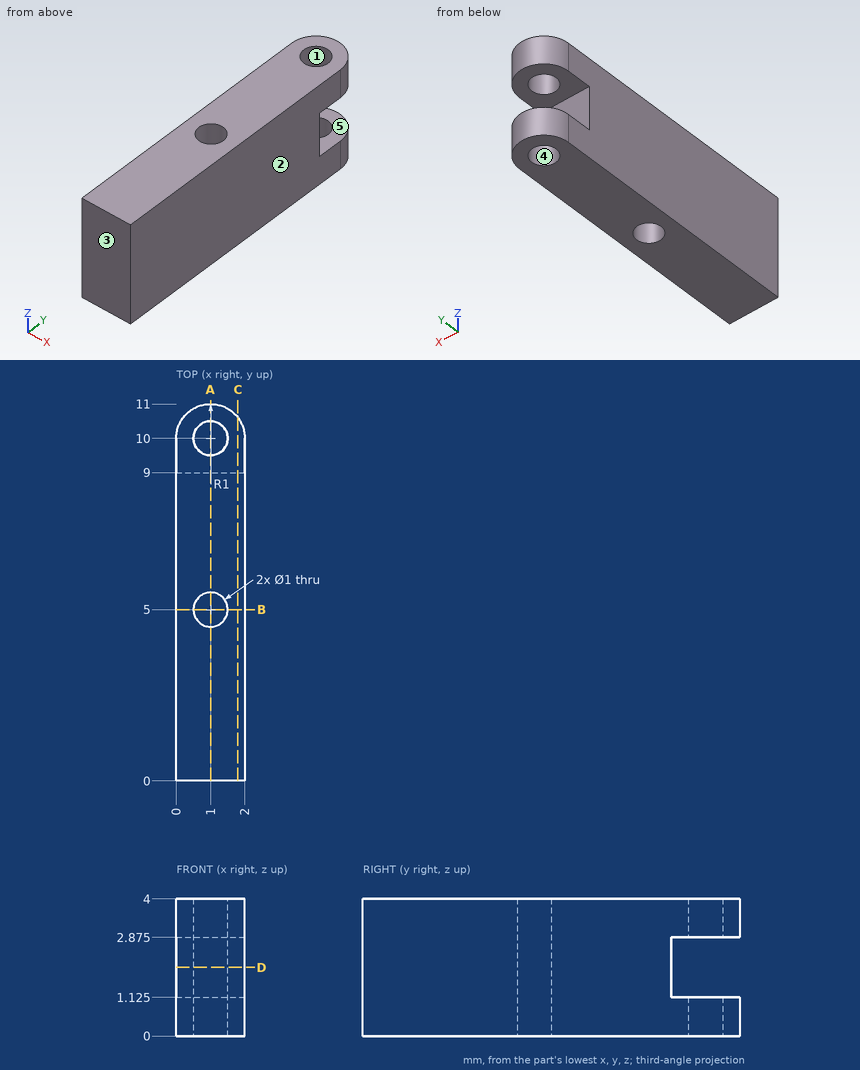
Drawing for the job (mm, zero at the part's lowest x, y, z). A direction names the side the tool comes from. Round coordinates to 2 decimals unless told otherwise and drop trailing zeros. Loops run counter-clockwise (first coordinate to the right, second up) from the corner with the lowest first, then second, coordinate; pieces in that order, holes last.
1. Wall check: probe 1 along Y at (x, z) = (1, 3.15); probe 2 along Y at (x, z) = (1, 1.3); probe 3 along X at (y, z) = (10, 0.35). Give the ranges that are in metal, low to high.
Check values:
probe 1: y = 0 to 4.5, 5.5 to 9.5, 10.5 to 11
probe 2: y = 0 to 4.5, 5.5 to 9
probe 3: x = 0 to 0.5, 1.5 to 2
2. Band-saw the part on D-D, the plane z = 2. List the corners of the cut face in (x, y), and give its area (3 significant figures).
Check values:
outline: (0, 0) - (2, 0) - (2, 9) - (0, 9) - close; hole circle Ø1 at (1, 5)
area: 17.2 mm2
3. Band-saw the part on B-B, the plane y = 5. List the corners of the cut face in (x, z).
Check values:
outline: (0, 0) - (0.5, 0) - (0.5, 4) - (0, 4) - close; (1.5, 0) - (2, 0) - (2, 4) - (1.5, 4) - close
4. Band-saw the part on A-A, the plane x = 1. List the corners of the cut face in (y, z) (3 decimals).
Check values:
outline: (0, 0) - (4.5, 0) - (4.5, 4) - (0, 4) - close; (5.5, 0) - (9.5, 0) - (9.5, 1.125) - (9, 1.125) - (9, 2.875) - (9.5, 2.875) - (9.5, 4) - (5.5, 4) - close; (10.5, 0) - (11, 0) - (11, 1.125) - (10.5, 1.125) - close; (10.5, 2.875) - (11, 2.875) - (11, 4) - (10.5, 4) - close
5. Tool access for the marked faces 4 and 5: list every direction of +Z, -Z, +X, -X, +Y, -Y with a clear straight run to the whole face (end or side of a thin tool).
Check values:
face 4: +Z, -Z
face 5: +X, -X, +Y
6. Mould opens along X. For the marked faces 1, 2 and 3 say: +X half, -X half, draft (parallel to the pull), parting line (faces both ways), or undercut.
Check values:
face 1: undercut
face 2: +X half
face 3: draft
7. Band-saw the part on C-C, the plane x = 1.8. List the corners of the cut face in (y, z) (3 decimals).
Check values:
outline: (0, 0) - (10.6, 0) - (10.6, 1.125) - (9, 1.125) - (9, 2.875) - (10.6, 2.875) - (10.6, 4) - (0, 4) - close
